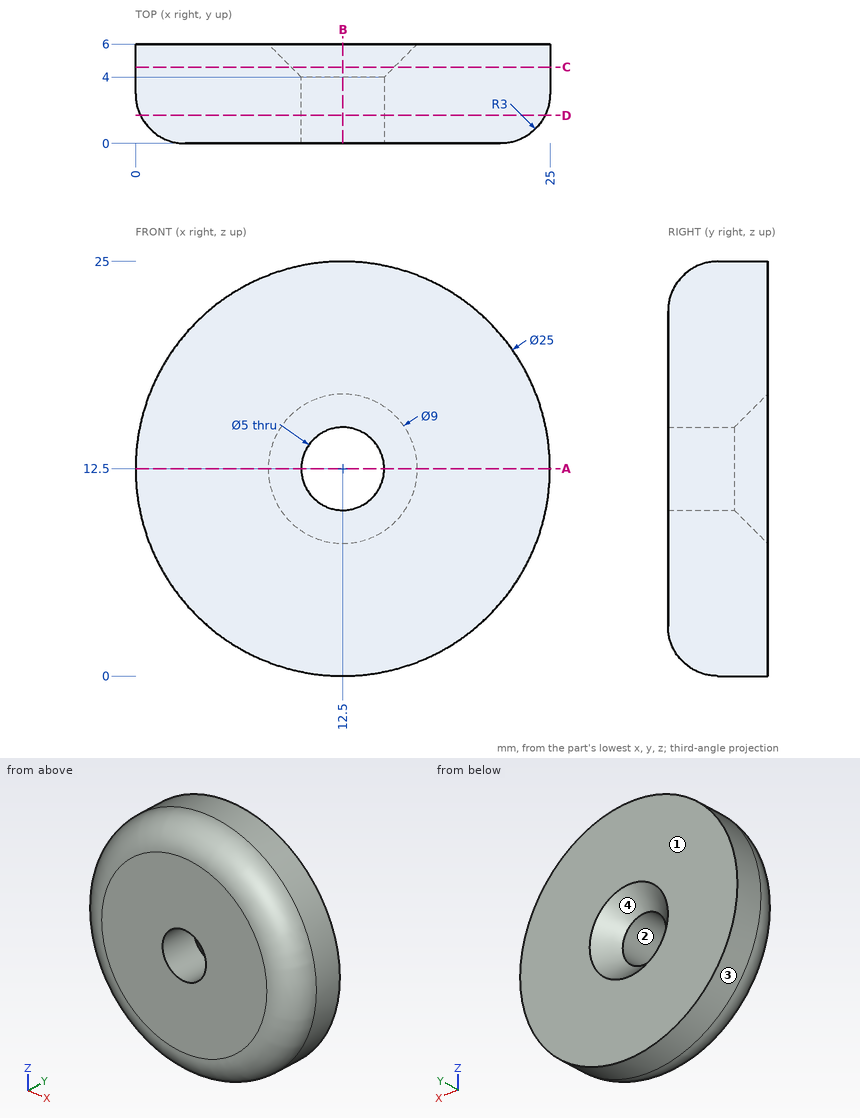
Source: three-view drawing plus pictorial views. Frame: mm from the lowest corner of the part. Give positions to 0.01 mm unless a question says otherwise; leave off trailing zeros. Order: outer loops, then holes, each group sorted by start corner. A loop starts at its lowest first (then second) coordinate and runs counter-clockwise, first axis right, second up. Notation, with made-up numbers: (79.5, 1.25) - (108.5, 1.25) arc R31 cw to (108.5, 34.25) - close; hole circle Ø7 at (36, -5). An arc over 180 degrees is marked (long way). Answer as a JSON object with one key per item and string values. Group by question number.
Q1. Cut plane A-A, the plane z = 12.5. Output: boundary loops of the cut face in (x, y).
Q2. Cut plane B-B, the plane x = 12.5. Output: boundary loops of the cut face in (y, z), then the cut area to 3 significant figures.
Q3. Line query: probe 1 along Z at (x, y) = (12.5, 3.1); probe 2 along Z at (x, y) = (12.5, 1.1); probe 3 along X at (y, z) = (3.55, 10.25). Output: solid intervals per line, ascending.
Q4. Cut plane D-D, the plane y = 1.7. Output: boundary loops of the cut face in (x, z), then the cut area to 3 significant figures.
Q5. Mould query, pull axis X, two halves, no side actions, for the marked faces 1, 2, 3 and 4. Classes: pulls with the +X half, pulls with the -X half, needs draft (parallel to the pull), parting line crosses it, or undercut.
Q6. First-contact query: pin 1 Ø2 at (y, z) = (5, 9.5) entering from -X; pin 2 Ø3 at (x, y) = (4, 4) entering from +Z; pin 3 Ø2 at (y, z) = (5, 16) entering from +X. Flat tips, straight axial feed; report the tip coordinate or a pass-through.
Q7. Cut plane C-C, the plane y = 4.6. Output: boundary loops of the cut face in (x, z), then the cut area to 3 significant figures.
Results:
{
 "1": {"outline": "(0, 3) arc R3 ccw to (3, 0) - (10, 0) - (10, 4) - (8, 6) - (0, 6) - close; (15, 0) - (22, 0) arc R3 ccw to (25, 3) - (25, 6) - (17, 6) - (15, 4) - close"},
 "2": {"outline": "(0, 3) arc R3 ccw to (3, 0) - (6, 0) - (6, 8) - (4, 10) - (0, 10) - close; (0, 15) - (4, 15) - (6, 17) - (6, 25) - (3, 25) arc R3 ccw to (0, 22) - close", "area": "112 mm^2"},
 "3": {"probe 1": "0 to 10, 15 to 25", "probe 2": "0.68 to 10, 15 to 24.32", "probe 3": "0.2 to 11.41, 13.59 to 24.8"},
 "4": {"outline": "circle Ø24.41 at (12.5, 12.5); hole circle Ø5 at (12.5, 12.5)", "area": "448 mm^2"},
 "5": {"face 1": "needs draft", "face 2": "undercut", "face 3": "parting line crosses it", "face 4": "undercut"},
 "6": {"pin 1": "x = 0.16", "pin 2": "z = 22.86", "pin 3": "x = 24.75"},
 "7": {"outline": "circle Ø25 at (12.5, 12.5); hole circle Ø6.2 at (12.5, 12.5)", "area": "461 mm^2"}
}
